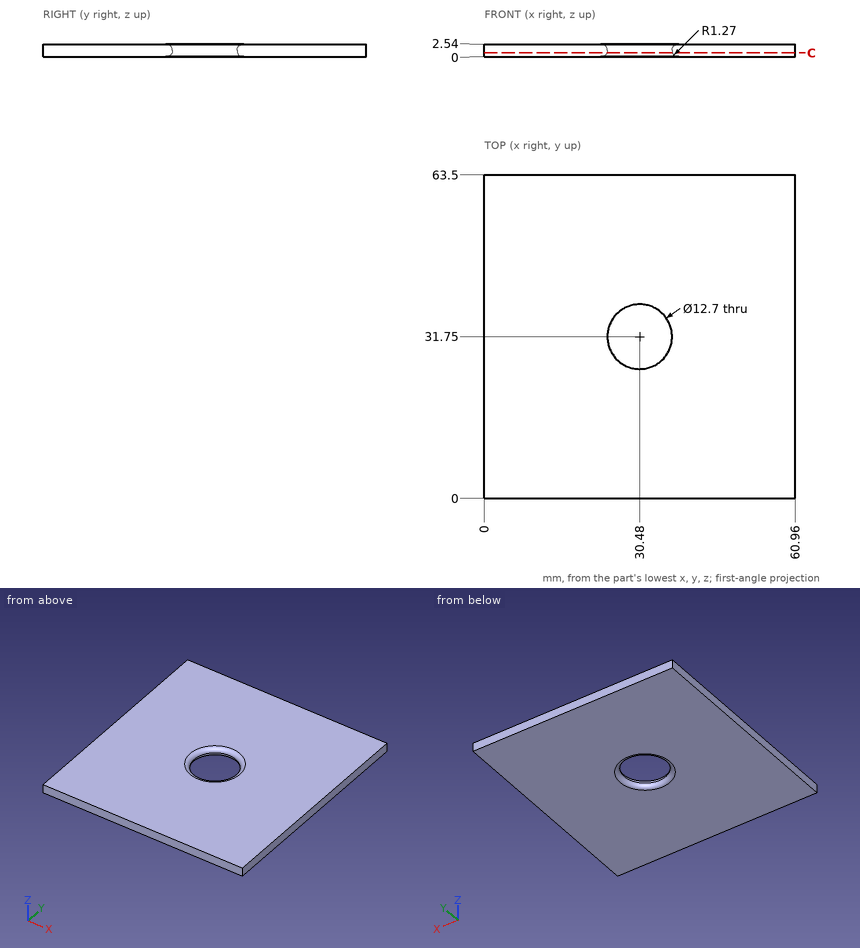
Input: dimensioned drawing with shaded views. Units: mm. Origin: part minimum x, y, z. Give positions to 0.01 mm unless a question says otherwise; leave off trailing zeros. Write each loop counter-clockwise with the first axis right and the second up, starting at its lowest first coordinate (ties: lowest second). Pieces come first, ordered by that corner, then holes.
Q1. Material intervals for probe 1 along Y at (x, z) = (30.48, 1.35); probe 2 along X at (y, z) = (35.5, 1.4); probe 3 along X at (y, z) = (28.5, 0.45), sorted ascending.
Q2. First-contact query: P1, Ø7.5, axis at x = 30.48, y = 31.75, coming from the +Z side; P2, Ø2, axis at x = 20.5, y = 40.5, coming from the -Z side. Flat tips, straight axial feed; report the tip coordinate or a pass-through.
Q3. Section C-C, the plane z = 0.8. Output: boundary loops of the cut face in (x, y), plus the area to 3 significant figures.
Filled in:
1. probe 1: y = 0 to 25.4, 38.1 to 63.5
1. probe 2: x = 0 to 25.35, 35.61 to 60.96
1. probe 3: x = 0 to 24.68, 36.28 to 60.96
2. P1: passes through
2. P2: stops at z = 0
3. outline: (0, 0) - (60.96, 0) - (60.96, 63.5) - (0, 63.5) - close; hole circle Ø12.88 at (30.48, 31.75)
3. area: 3,740 mm2
